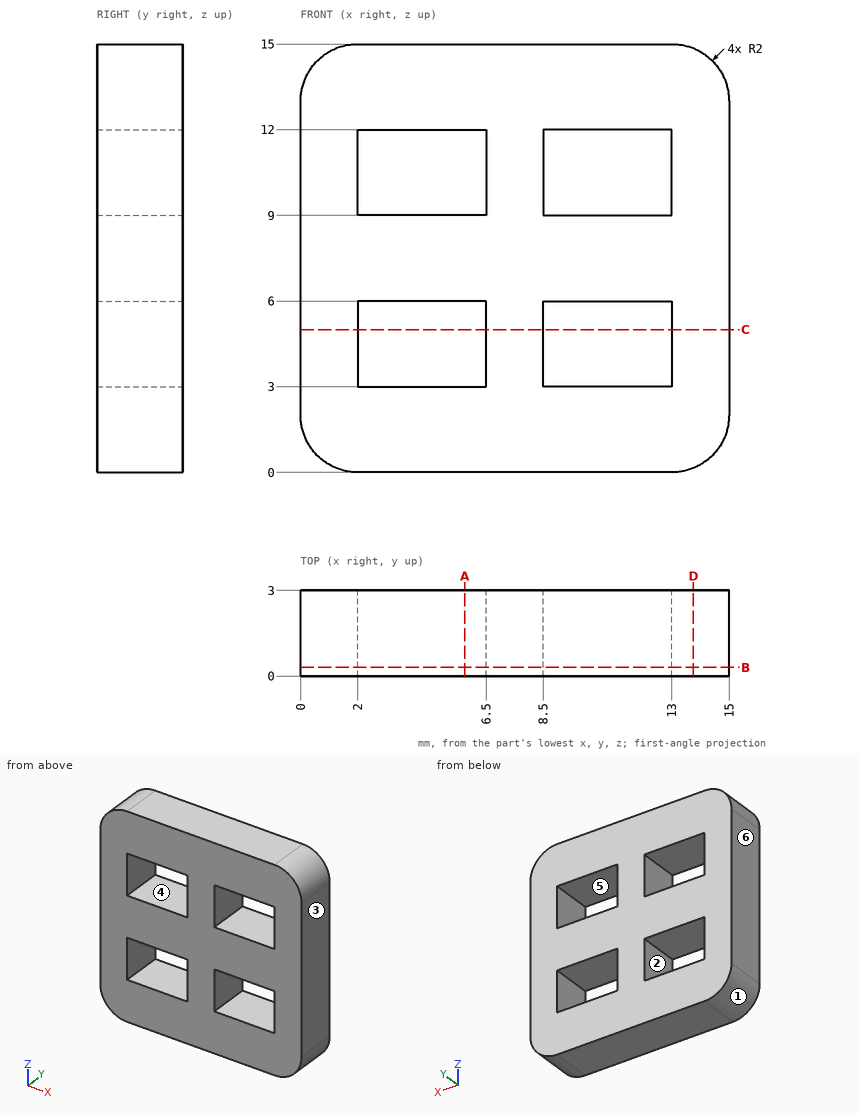
Geometry check sheet. Reference: drawing and pictorial views, mm from the part's lowest x, y, z. A direction names the side the tool comes from. Round coordinates to 2 decimals unless told otherwise and drop trailing zeros. Order: outer loops, then holes, each group sorted by start corner. A loop starts at its lowest first (then second) coordinate and runs counter-clockwise, first axis right, second up. Notation, with made-up numbers: (-38, -20) - (-28, -20) arc R13 ccw to (-28, -13) - close; hole circle Ø4 at (23, 3.5). An arc over 180 degrees is marked (long way). Use a Markdown table: item, result. Add a question column.
1) Thickness scan on line 1 along X through (y, z) = (0.3, 10.5); line 2 along Z through (x, y) = (3.25, 1.65); line 3 along X through (y, z) = (0.85, 14). Record the ranges inside material, lowest first.
2) Section check C-C (z = 5). Record the cut outline in (x, y), then the cut area to 3 significant figures.
3) Mould release check, pull along X, two halves, no side actions. Record for the marked faces 3, 4, 5 and 6: released by +X, released by -X, zero draft, split by the parting line, or undercut.
4) Section check A-A (x = 5.75). Record the cut outline in (y, z), then the cut area to 3 significant figures.
5) Section check B-B (y = 0.3). Record the cut outline in (x, z).
6) Section check D-D (x = 13.75). Record the cut outline in (y, z), then the cut area to 3 significant figures.
7) Set-up check for the marked faces 1 and 2: record each of +Z, -Z, +X, -X, +Y, -Y from which the full face is reachable in a straight line by a thin tool's end or side.
Established:
| question | item | result |
|---|---|---|
| 1 | line 1 | 0 to 2, 6.5 to 8.5, 13 to 15 |
| 1 | line 2 | 0 to 3, 6 to 9, 12 to 15 |
| 1 | line 3 | 0.27 to 14.73 |
| 2 | outline | (0, 0) - (2, 0) - (2, 3) - (0, 3) - close; (6.5, 0) - (8.5, 0) - (8.5, 3) - (6.5, 3) - close; (13, 0) - (15, 0) - (15, 3) - (13, 3) - close |
| 2 | area | 18.0 mm2 |
| 3 | face 3 | released by +X |
| 3 | face 4 | undercut |
| 3 | face 5 | undercut |
| 3 | face 6 | released by -X |
| 4 | outline | (0, 0) - (3, 0) - (3, 3) - (0, 3) - close; (0, 6) - (3, 6) - (3, 9) - (0, 9) - close; (0, 12) - (3, 12) - (3, 15) - (0, 15) - close |
| 4 | area | 27.0 mm2 |
| 5 | outline | (0, 2) arc R2 ccw to (2, 0) - (13, 0) arc R2 ccw to (15, 2) - (15, 13) arc R2 ccw to (13, 15) - (2, 15) arc R2 ccw to (0, 13) - close; hole (2, 3) - (6.5, 3) - (6.5, 6) - (2, 6) - close; hole (2, 9) - (6.5, 9) - (6.5, 12) - (2, 12) - close; hole (8.5, 3) - (13, 3) - (13, 6) - (8.5, 6) - close; hole (8.5, 9) - (13, 9) - (13, 12) - (8.5, 12) - close |
| 6 | outline | (0, 0.15) - (3, 0.15) - (3, 14.85) - (0, 14.85) - close |
| 6 | area | 44.1 mm2 |
| 7 | face 1 | -Z, -X, +Y, -Y |
| 7 | face 2 | +Y, -Y |
